Part model, mm, in its own coordinate system. Face numbers are marked on the shaded views. A direction names the side the tool comes from. Give positions to 0.01 mm unless a question says otherwise; leave off trailing zeros. Write each loop counter-clockwise with the first axis right and the second up, starting at its lowest first coordinate (ties: lowest second). Pieces come first, ordered by that corner, then holes. Notation, with made-up numbers: M 81,7 L 115,7 A21 cw 115,25 Z; hole C -28.75,-25.5 d2. An arc over 180 degrees is marked long. Answer as CSV lines item,"result". Start each with the question number.
Item 1: 3-axis set-ups, long thin cutter, end or side, ignore diameter. For the marked faces 1, 2 and 3: which of +Z, -Z, +X, -X, +Y, -Y reach the whole face in a straight line?
Item 2: Pin check, flat tips, straight feed: pin 1 (0.6 mm diameter, centred on y = 0, z = 0, fed in from -X); pin 2 (1 mm diameter, centred on y = -0.5, z = -2, fed in from +X); pin 3 (1.5 mm diameter, centred on x = 1.5, z = -0.5, fed in from -Y). Stop position of each tip, or through.
Item 3: Band-saw the part on C-C, the plane x = -0.5. List the corners of the cut face in (y, z).
Item 4: Wall check: L1, parallel to X at y = 1, z = 1.5; L2, parallel to X at y = -0.65, z = 0.25; L3, parallel to Y at x = -2, z = 0.05. Give the ranges that are in metal, low to high. Write a range as from..to.
Item 5: Band-saw the part on B-B, the plane x = 3. List the corners of the cut face in (y, z), then the cut area to 3 significant figures.
from build123d import *

# Parameters (mm, degrees)
CUT_EXTRUDE1_DEPTH = 1.1


with BuildPart() as part:
    # Sketch1 → Revolve1 (revolve)
    with BuildSketch(Plane.XY):
        with BuildLine():
            Line((5.7465, 1.25), (0.125, 1.25))
            ThreePointArc((0.125, 1.25), (0.036611652, 1.286611652), (0, 1.375))
            Line((0, 1.375), (0, 2.25))
            Line((0, 2.25), (-2.375, 2.25))
            ThreePointArc((-2.375, 2.25), (-2.463388348, 2.213388348), (-2.5, 2.125))
            Line((-2.5, 2.125), (-2.5, 0))
            Line((-2.5, 0), (6, 0))
            Line((6, 0), (6, 0.9965))
            Line((6, 0.9965), (5.7465, 1.25))
        make_face()
    revolve(axis=Axis((-2.5, 0, 0), (1, 0, 0)))

    # Sketch2 → Cut-Extrude1 (cut)
    with BuildSketch(Plane.ZY.offset(2.5)):
        Polygon((1.025, 0.591784026), (0, 1.183568052), (-1.025, 0.591784026), (-1.025, -0.591784026), (0, -1.183568052), (1.025, -0.591784026), align=None)
    extrude(amount=-CUT_EXTRUDE1_DEPTH, mode=Mode.SUBTRACT)


solid = part.part
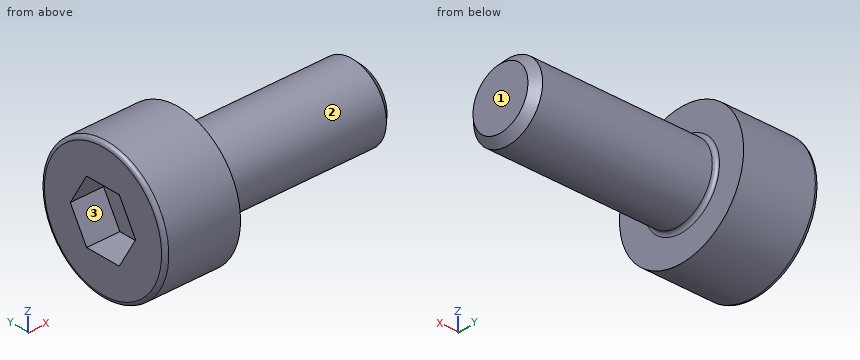
Output:
1,face 1,"+Z, -Z, +X, +Y, -Y"
1,face 2,"+X"
1,face 3,"-X"
2,pin 1,"x = -1.4"
2,pin 2,"x = 0"
2,pin 3,"y = -1.25"
3,outline,"C 0,0 d4.5"
4,L1,"-2.5..0"
4,L2,"-1.4..6"
4,L3,"-2.25..-1.15, 1.15..2.25"
5,outline,"C 0,0 d2.5"
5,area,"4.91 mm²"
